The listing builds one solid part. Answer for the finished solid, in the listing's coordinates (mm). Coordinates: 2 decimals unless noted, no trailing zeros. Order: outer loops, then holes, each group sorted by start corner. A loop starts at its lowest first (then second) coordinate and runs counter-clockwise, first axis right, second up. Notation, with made-up numbers: (77.25, -16.5) - (104.25, -16.5) arc R6 ccw to (104.25, -9.5) - close; hole circle Ø6 at (4.25, 9.5). An arc over 180 degrees is marked (long way). Use a Markdown table: item, result. Add a question column.
Item 1: A flat-ended cylindrical pin translates along its axis: P1, Ø0.9, axis at x = -46, z = 1, coming from the -Y side. Find the tip coordinate at first contact, or state that the pin passes through.
Item 2: Find the intervals of material crossed by line 1 along X through (y, z) = (49, 1.35); line 2 along Y through (x, z) = (-60, 1.6); line 3 along Y through (x, z) = (-44, 2), in increasing order.
Item 3: The part is cut by section A-A, the plane z = 2.55. Give the vertices of the cut face in (x, y).
from build123d import *

# Parameters (mm, degrees)
SKETCH1_W           = 203
SKETCH1_H           = 150
BOSS_EXTRUDE1_DEPTH = 3
SKETCH2_W           = 15
SKETCH2_H           = 15
CUT_EXTRUDE1_DEPTH  = 127.238860895
SKETCH3_W           = 30
SKETCH3_H           = 3
CUT_EXTRUDE2_DEPTH  = 10


with BuildPart() as part:
    # Sketch1 → Boss-Extrude1 (new body)
    with BuildSketch(Plane.XY):
        Rectangle(SKETCH1_W, SKETCH1_H)
    extrude(amount=BOSS_EXTRUDE1_DEPTH)

    # Sketch2 → Cut-Extrude1 (cut, through all)
    with BuildSketch(Plane.XY.offset(3)):
        with Locations((-57.5, 47.5)):
            Rectangle(SKETCH2_W, SKETCH2_H)
        with Locations((57.5, 47.5)):
            Rectangle(SKETCH2_W, SKETCH2_H)
        with Locations((0, 47.5)):
            Rectangle(SKETCH2_W, SKETCH2_H)
    extrude(amount=-CUT_EXTRUDE1_DEPTH, mode=Mode.SUBTRACT)

    # Sketch3 → Cut-Extrude2 (cut)
    with BuildSketch(Plane.XY.offset(3)):
        with Locations((-48.5, -73.5)):
            Rectangle(SKETCH3_W, SKETCH3_H)
        with Locations((51.5, -73.5)):
            Rectangle(SKETCH3_W, SKETCH3_H)
    extrude(amount=-CUT_EXTRUDE2_DEPTH, mode=Mode.SUBTRACT)


solid = part.part
Solution:
| question | item | result |
|---|---|---|
| 1 | P1 | stops at y = -72 |
| 2 | line 1 | x = -101.5 to -65, -50 to -7.5, 7.5 to 50, 65 to 101.5 |
| 2 | line 2 | y = -72 to 40, 55 to 75 |
| 2 | line 3 | y = -72 to 75 |
| 3 | outline | (-101.5, -75) - (-63.5, -75) - (-63.5, -72) - (-33.5, -72) - (-33.5, -75) - (36.5, -75) - (36.5, -72) - (66.5, -72) - (66.5, -75) - (101.5, -75) - (101.5, 75) - (-101.5, 75) - close; hole (-65, 40) - (-50, 40) - (-50, 55) - (-65, 55) - close; hole (-7.5, 40) - (7.5, 40) - (7.5, 55) - (-7.5, 55) - close; hole (50, 40) - (65, 40) - (65, 55) - (50, 55) - close |
